from build123d import *

# Parameters (mm, degrees)
SKETCH2_W                = 50
SKETCH2_H                = 65
SKETCH2_R                = 1.6
SKETCH2_W_2              = 9.2
SKETCH2_H_2              = 5
BOSS_EXTRUDE1_DEPTH      = 5
SKETCH3_W                = 9.2
SKETCH3_H                = 5
BOSS_EXTRUDE2_DEPTH      = 25
BOSS_EXTRUDE2_DEPTH_BACK = 5
SKETCH4_R                = 1.6
CUT_EXTRUDE1_DEPTH       = 32.65
SKETCH5_W                = 9.2
SKETCH5_H                = 18.65
BOSS_EXTRUDE3_DEPTH      = 5
FILLET1_R                = 1


with BuildPart() as part:
    # Sketch2 → Boss-Extrude1 (new body)
    with BuildSketch(Plane.XY):
        Rectangle(SKETCH2_W, SKETCH2_H)
        with Locations((-13.25, -29.25)):
            Circle(SKETCH2_R, mode=Mode.SUBTRACT)
        with Locations((13.25, -29.25)):
            Circle(SKETCH2_R, mode=Mode.SUBTRACT)
        with Locations((13.25, 29.25)):
            Circle(SKETCH2_R, mode=Mode.SUBTRACT)
        with Locations((-13.25, 29.25)):
            Circle(SKETCH2_R, mode=Mode.SUBTRACT)
        with Locations((29.6, -27)):
            Rectangle(SKETCH2_W_2, SKETCH2_H_2)
        with BuildLine():
            Line((25, -29.5), (25, -24.5))
            Line((25, -24.5), (-25, -24.5))
            Line((-25, -24.5), (-25, -29.5))
            Line((-25, -29.5), (-14.830348063, -29.5))
            ThreePointArc((-14.830348063, -29.5), (-13.375385604, -27.65492055), (-11.65, -29.25))
            ThreePointArc((-11.65, -29.25), (-11.65492055, -29.375385604), (-11.669651937, -29.5))
            Line((-11.669651937, -29.5), (11.669651937, -29.5))
            ThreePointArc((11.669651937, -29.5), (13.124614396, -27.65492055), (14.85, -29.25))
            ThreePointArc((14.85, -29.25), (14.84507945, -29.375385604), (14.830348063, -29.5))
            Line((14.830348063, -29.5), (25, -29.5))
        make_face()
        with Locations((-29.6, -27)):
            Rectangle(SKETCH2_W_2, SKETCH2_H_2)
        with BuildLine():
            Line((25, -32.5), (25, -29.5))
            Line((25, -29.5), (14.830348063, -29.5))
            ThreePointArc((14.830348063, -29.5), (13.25, -30.85), (11.669651937, -29.5))
            Line((11.669651937, -29.5), (-11.669651937, -29.5))
            ThreePointArc((-11.669651937, -29.5), (-13.25, -30.85), (-14.830348063, -29.5))
            Line((-14.830348063, -29.5), (-25, -29.5))
            Line((-25, -29.5), (-25, -32.5))
            Line((-25, -32.5), (25, -32.5))
        make_face()
    extrude(amount=BOSS_EXTRUDE1_DEPTH)

    # Sketch3 → Boss-Extrude2 (add, two sides)
    with BuildSketch(Plane(origin=(0, 0, 0), x_dir=(-1, 0, 0), z_dir=(0, 0, -1))) as boss_extrude2_sk:
        with Locations((-29.6, -27)):
            Rectangle(SKETCH3_W, SKETCH3_H)
        with Locations((-29.6, -3.35)):
            Rectangle(SKETCH3_W, SKETCH3_H)
        with Locations((29.6, -27)):
            Rectangle(SKETCH3_W, SKETCH3_H)
        with Locations((29.6, -3.35)):
            Rectangle(SKETCH3_W, SKETCH3_H)
    extrude(amount=BOSS_EXTRUDE2_DEPTH)
    extrude(boss_extrude2_sk.sketch, amount=-BOSS_EXTRUDE2_DEPTH_BACK)

    # Sketch4 → Cut-Extrude1 (cut, through all)
    with BuildSketch(Plane(origin=(0, -0.85, 0), x_dir=(1, 0, 0), z_dir=(0, 1, 0))):
        with Locations((27.6, 17.5)):
            Circle(SKETCH4_R)
        with Locations((-27.6, 17.5)):
            Circle(SKETCH4_R)
    extrude(amount=-CUT_EXTRUDE1_DEPTH, mode=Mode.SUBTRACT)

    # Sketch5 → Boss-Extrude3 (add)
    with BuildSketch(Plane.XY.offset(5)):
        with Locations((-29.6, -15.175)):
            Rectangle(SKETCH5_W, SKETCH5_H)
        with Locations((29.6, -15.175)):
            Rectangle(SKETCH5_W, SKETCH5_H)
    extrude(amount=-BOSS_EXTRUDE3_DEPTH)

    # Fillet1
    fillet1_edges = [part.edges().sort_by_distance(p)[0] for p in [
        (-29.6, -29.5, 5),
        (0, -32.5, 5),
        (29.6, -29.5, 5),
        (0, 32.5, 5),
        (-29.6, -0.85, 5),
        (29.6, -0.85, 5),
    ]]
    fillet(fillet1_edges, radius=FILLET1_R)


solid = part.part
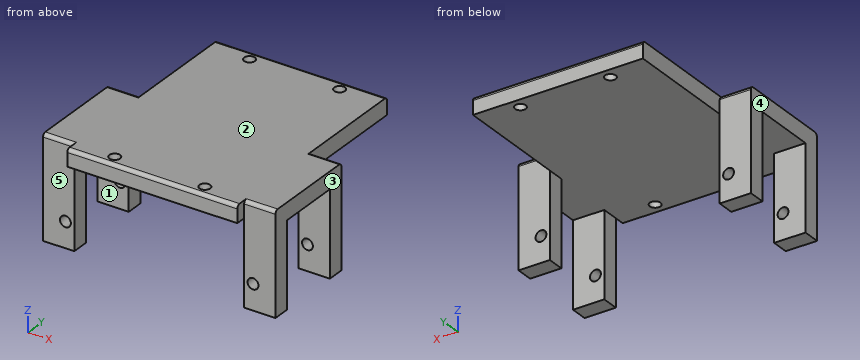
Model file for the job. Use its own axes, mm. Face numbers are marked on the shaded views. A direction names the side the tool comes from. Give positions to 0.01 mm unless a question says otherwise; leave off trailing zeros. Write each loop counter-clockwise with the first axis right and the second up, starting at its lowest first coordinate (ties: lowest second). Pieces come first, ordered by that corner, then holes. Notation, with made-up numbers: M 7,10.25 L 44,10.25 A26 ccw 44,42.25 Z; hole C 11.5,-9.75 d4. An arc over 180 degrees is marked long. One line per item, written item: value. Start each with the question number.
Q1. Saw through at D-D, the plane x = 13.25. Write the cut outline in (y, z).
Q2. Saw through at B-B, the plane z = -1. Write the cut outline in (x, y).
Q3. Probe probe 1 along X at (y, z) = (-29.25, 1.95); probe 2 along X at (y, z) = (-28.5, -17.5); probe 3 along Y at (x, z) = (-13.25, 1.45). List the from-to ranges inside material, lowest first. Write a range as [from, to].
Q4. Drop flat-ended pins along their axis: pin 1 Ø1 at (x, y) = (2.5, 11.5) entering from -Z; pin 2 Ø3 at (x, z) = (-29.5, -6.5) entering from +Y; pin 3 Ø4.5 at (x, z) = (-29.5, -14) entering from -Y. Give the stop position or say it passes through.
Q5. Saw through at A-A, the plane x = -27.6. Write the cut outline in (y, z).
Q6. Two-plate mould, pull along X, no slides. Class the marked faces 3, 4 and 5: +X half, -X half, draft (parallel to the pull), parting line (faces both ways), or undercut.
Q7. 3-axis set-ups, long thin cutter, end or side, ignore diameter. For the marked faces 1 and 2: which of +Z, -Z, +X, -X, +Y, -Y reach the whole face in a straight line?
Q8. Saw through at C-C, the plane z = -17.5. State how many separate pieces and enclosed holes the cut face has, plus the area to 3 significant figures.
Output values:
1. outline: M -32.5,0 L -30.85,0 L -30.85,5 L -31.5,5 A1 ccw -32.5,4 Z; M -27.65,0 L 27.65,0 L 27.65,5 L -27.65,5 Z; M 30.85,0 L 32.5,0 L 32.5,4 A1 ccw 31.5,5 L 30.85,5 Z
2. outline: M -34.2,-29.5 L -25,-29.5 L -25,-24.5 L -34.2,-24.5 Z; M -34.2,-5.85 L -25,-5.85 L -25,-0.85 L -34.2,-0.85 Z; M 25,-29.5 L 34.2,-29.5 L 34.2,-24.5 L 25,-24.5 Z; M 25,-5.85 L 34.2,-5.85 L 34.2,-0.85 L 25,-0.85 Z
3. probe 1: x = [-34.2, -14.85], [-11.65, 11.65], [14.85, 34.2]
3. probe 2: x = [-34.2, -29.2], [-26, -25], [25, 26], [29.2, 34.2]
3. probe 3: y = [-32.5, -30.85], [-27.65, 27.65], [30.85, 32.5]
4. pin 1: stops at z = 0
4. pin 2: stops at y = -0.85
4. pin 3: stops at y = -29.5
5. outline: M -29.5,-25 L -24.5,-25 L -24.5,-19.1 L -29.5,-19.1 Z; M -29.5,-15.9 L -24.5,-15.9 L -24.5,0 L -5.85,0 L -5.85,-15.9 L -0.85,-15.9 L -0.85,4 A1 ccw -1.85,5 L -28.5,5 A1 ccw -29.5,4 Z; M -5.85,-25 L -0.85,-25 L -0.85,-19.1 L -5.85,-19.1 Z
6. face 3: +X half
6. face 4: -X half
6. face 5: draft
7. face 1: -Z, +X, -X
7. face 2: +Z, +X, -X, +Y, -Y
8. separate pieces: 8
8. enclosed holes: 0
8. area: 120 mm²
